```python
from build123d import *

# Parameters (mm, degrees)
F1_DEPTH = 2000
F2_T     = -1.6
F3_R     = 130
F3_W     = 240
F3_H     = 400
F4_DEPTH = 60.001


with BuildPart() as f1:
    # F0 (on Front) → F1 (new body)
    with BuildSketch(Plane.XZ):
        Polygon((0, 60), (0, 0), (1010, 0), (1010, 60), (460, 60), (460, 110), (400, 110), (400, 60), align=None)
    extrude(amount=F1_DEPTH)

    # F2
    f2_openings = [f1.faces().sort_by_distance(p)[0] for p in [
        (505, -1000, 0),
        (501.462264, -2000, 32.59434),
        (501.462264, 0, 32.59434),
    ]]
    offset(amount=F2_T, openings=f2_openings, kind=Kind.INTERSECTION)

    # F3 (on face) → F4 (cut, through all)
    with BuildSketch(Plane.XY.offset(60)):
        with Locations((200, -1000)):
            Circle(F3_R)
        with Locations((200, -430)):
            Rectangle(F3_W, F3_H)
        with Locations((200, -1570)):
            Rectangle(F3_W, F3_H)
    extrude(amount=-F4_DEPTH, mode=Mode.SUBTRACT)


solid = f1.part
```
Design review of the part built by this model. Coordinates are the model's own, in mm. A direction names the side the tool comes from. Round coordinates to 2 decimals unless told otherwise and drop trailing zeros. Write each loop counter-clockwise with the first axis right and the second up, starting at its lowest first coordinate (ties: lowest second). Pieces come first, ordered by that corner, then holes.
Item 1: We need section A-A on x = 200. Write out the cut boundary in (y, z).
Item 2: We need section D-D on y = -560.5. Write out the cut boundary in (x, z), and give its area (3 significant figures).
Item 3: For faces 4 (the flat face through (503, 0, 59)), 5 (the flat face through (460, -986, 85)), 6 (the flat face through (1008.4, -986, 29)), 7 (the flat face through (400, -986, 85)), list the 3-axis set-ups (+Z, -Z, +X, -X, +Y, -Y) from which the entire face can be reached by the end or side of a thin tool; tool diameter is ignored.
Item 4: The part is to be moulded in two halves that separate along X. For faces 1 (the flat face through (739, -986, 60)), 2 (the flat face through (1.6, -986, 30)), 3 (the flat face through (1010, -986, 30)), say which applies: +X half, -X half, draft (parallel to the pull), parting line (faces both ways), or undercut.
Item 5: Clearance check with flat-ended pins moving along their axes: pin 1 Ø1 at (y, z) = (-267, 61) entering from +X; pin 2 Ø12 at (x, y) = (162.5, -696.5) entering from +Z. State where each tip first meets the part, or that it passes through.
Item 6: We need section B-B on y = -1000. Write out the cut boundary in (x, z).
Item 7: We need section C-C on z = 34. Write out the cut boundary in (x, y).
Item 8: For probe 1 along Y at (x, z) = (200, 59); probe 2 along X at (y, z) = (-1830.5, 94); probe 3 along X at (y, z) = (-1644.5, 35.5), list the stretches that pass through material, from the lowest coordinate up.
Returned:
1. outline: (-2000, 58.4) - (-1770, 58.4) - (-1770, 60) - (-2000, 60) - close; (-1370, 58.4) - (-1130, 58.4) - (-1130, 60) - (-1370, 60) - close; (-870, 58.4) - (-630, 58.4) - (-630, 60) - (-870, 60) - close; (-230, 58.4) - (0, 58.4) - (0, 60) - (-230, 60) - close
2. outline: (0, 0) - (1.6, 0) - (1.6, 58.4) - (80, 58.4) - (80, 60) - (0, 60) - close; (320, 58.4) - (401.6, 58.4) - (401.6, 108.4) - (458.4, 108.4) - (458.4, 58.4) - (1008.4, 58.4) - (1008.4, 0) - (1010, 0) - (1010, 60) - (460, 60) - (460, 110) - (400, 110) - (400, 60) - (320, 60) - close
2. area: 1,580 mm2
3. face 4: +Z, -Z, +X, -X, +Y
3. face 5: +Z, +X, +Y, -Y
3. face 6: -Z, +Y, -Y
3. face 7: +Z, -X, +Y, -Y
4. face 1: draft
4. face 2: undercut
4. face 3: +X half
5. pin 1: stops at x = 460
5. pin 2: stops at z = 60
6. outline: (0, 0) - (1.6, 0) - (1.6, 58.4) - (70, 58.4) - (70, 60) - (0, 60) - close; (330, 58.4) - (401.6, 58.4) - (401.6, 108.4) - (458.4, 108.4) - (458.4, 58.4) - (1008.4, 58.4) - (1008.4, 0) - (1010, 0) - (1010, 60) - (460, 60) - (460, 110) - (400, 110) - (400, 60) - (330, 60) - close
7. outline: (0, -2000) - (1.6, -2000) - (1.6, 0) - (0, 0) - close; (1008.4, -2000) - (1010, -2000) - (1010, 0) - (1008.4, 0) - close
8. probe 1: y = -2000 to -1770, -1370 to -1130, -870 to -630, -230 to 0
8. probe 2: x = 400 to 401.6, 458.4 to 460
8. probe 3: x = 0 to 1.6, 1008.4 to 1010
